Source: CAD feature listing. Evaluate the final solid. Frame: model axes, mm. A direction names the side the tool comes from. Give positions to 0.01 mm unless a question says otherwise; leave off trailing zeros. Loops run counter-clockwise (first coordinate to the right, second up) from the corner with the lowest first, then second, coordinate; pieces in that order, holes last. Notation, with made-up numbers: M 60.5,-37.75 L 99.5,-37.75 A22 ccw 99.5,1.25 Z; hole C -12.5,-32 d3. An arc over 180 degrees is marked long. Write item = value, one per line.
from build123d import *

# Parameters (mm, degrees)
SKETCH1_R           = 25
SKETCH1_R_2         = 20
BOSS_EXTRUDE1_DEPTH = 15
SKETCH2_R           = 35
SKETCH2_R_2         = 25
BOSS_EXTRUDE2_DEPTH = 7.5
SKETCH3_W           = 5
SKETCH3_H           = 16.794369207
BOSS_EXTRUDE3_DEPTH = 7


with BuildPart() as part:
    # Sketch1 → Boss-Extrude1 (new body)
    with BuildSketch(Plane.XY):
        Circle(SKETCH1_R)
        Circle(SKETCH1_R_2, mode=Mode.SUBTRACT)
    extrude(amount=BOSS_EXTRUDE1_DEPTH)

    # Sketch2 → Boss-Extrude2 (add)
    with BuildSketch(Plane(origin=(0, 0, 0), x_dir=(-1, 0, 0), z_dir=(0, 0, -1))):
        Circle(SKETCH2_R)
        Circle(SKETCH2_R_2, mode=Mode.SUBTRACT)
    extrude(amount=-BOSS_EXTRUDE2_DEPTH)

    # Sketch3 → Boss-Extrude3 (add)
    with BuildSketch(Plane.XY):
        with Locations((0, 36.602815396)):
            Rectangle(SKETCH3_W, SKETCH3_H)
    extrude(amount=BOSS_EXTRUDE3_DEPTH)


solid = part.part
1. Reachability of faces 1 (the flat face through (-2.5, 40, 3)), 2 (the flat face through (2.5, 40, 3)), 3 (the cylindrical face through (23.846, 7.509, 11.198)), 4 (the flat face through (16.05, -12.22, 0)) from +Z, -Z, +X, -X, +Y, -Y: full face, straight path, thin tool, end or side. Return the list, or none.
Derived:
face_1 = +Z, -Z, -X, +Y
face_2 = +Z, -Z, +X, +Y
face_3 = +Z
face_4 = -Z, +X, -X, +Y, -Y
2. First-contact query: pin 1 Ø1 at (x, z) = (5, 3) entering from -Y; pin 2 Ø1 at (x, y) = (-27, 25) entering from +Z; pin 3 Ø1.5 at (x, y) = (1, 38) entering from +Z; pin 4 Ø8 at (x, y) = (-22.5, -13.5) entering from +Z. Flat tips, straight axial feed; report the tip coordinate or a pass-through.
Derived:
pin_1 = -34.71
pin_2 = through
pin_3 = 7
pin_4 = 15
3. Pull-direction query (Y, two-part tool) for faces 5 (the flat face through (0, 40, 7)), 6 (the cylindrical face through (-4.336, -19.524, 7.395)), 7 (the flat face through (0, 45, 3)); classes: +Y half, -Y half, draft (parallel to the pull), parting line (faces both ways), or undercut.
Derived:
face_5 = draft
face_6 = undercut
face_7 = +Y half
4. Material intervals for probe 1 along Y at (x, z) = (0, 11.25); probe 2 along Z at (x, y) = (20, 21.5); probe 3 along X at (y, z) = (-9, 11), sorted ascending. Write a range as from..to.
Derived:
probe_1 = -25..-20, 20..25
probe_2 = 0..7.5
probe_3 = -23.32..-17.86, 17.86..23.32
5. Cut plane B-B, the plane x = 0. Return the cut outline in (y, z), then the cut area to 3 significant figures.
Derived:
outline = M -35,0 L -20,0 L -20,15 L -25,15 L -25,7.5 L -35,7.5 Z; M 20,0 L 45,0 L 45,7 L 35,7 L 35,7.5 L 25,7.5 L 25,15 L 20,15 Z
area = 370 mm²
6. Cut plane D-D, the plane y = 13. Return the cut outline in (x, z), then the cut area to 3 significant figures.
Derived:
outline = M -32.5,0 L -15.2,0 L -15.2,15 L -21.35,15 L -21.35,7.5 L -32.5,7.5 Z; M 15.2,0 L 32.5,0 L 32.5,7.5 L 21.35,7.5 L 21.35,15 L 15.2,15 Z
area = 352 mm²
7. Cut plane A-A, the plane y = 0. Return the cut outline in (x, z), then the cut area to 3 significant figures.
Derived:
outline = M -35,0 L -20,0 L -20,15 L -25,15 L -25,7.5 L -35,7.5 Z; M 20,0 L 35,0 L 35,7.5 L 25,7.5 L 25,15 L 20,15 Z
area = 300 mm²
8. Cut plane C-C, the plane z = 2.75. Return the cut outline in (x, y), then the cut area to 3 significant figures.
Derived:
outline = M -2.5,34.91 A35 ccw long 2.5,34.91 L 2.5,45 L -2.5,45 Z; hole C 0,0 d40
area = 2,640 mm²
